Can you work these out from the model? Positions are in its coordinate system, mm. A direction names the side the tool comes from. Round coordinates to 2 decimals unless told otherwise and drop trailing zeros. Write each loop counter-clockwise with the first axis right and the second up, starting at its lowest first coordinate (ties: lowest second). Pieces come first, ordered by that corner, then holes. Notation, with made-up numbers: M 42.25,-39.5 L 91.25,-39.5 A21 ccw 91.25,-30.5 Z; hole C -35.75,-19.75 d9. An arc over 180 degrees is marked long. Answer as a JSON object with one key per item and string values. Group by question number.
1) Please list where these lines run through material, in increasing order: L1, parallel to Y at x = 0, z = 6.1; L2, parallel to Y at x = -2.5, z = 4; L3, parallel to X at y = 4.25, z = 7.5. Write a range as [from, to].
2) If we mould it in two halves opening along Y, with no side actions, what happens to faces 1 (the flat face through (0, -4, 8)), 2 (the flat face through (0, 4.75, 5)), 3 (the cylindrical face through (-0.75, 5.7, 5.97))? For each: +Y half, -Y half, draft (parallel to the pull), parting line (faces both ways), or undercut.
3) Suppose I cut it at A-A, the plane z = 7.5. Write out the boundary of the cut face in (x, y), and give its area (3 significant figures).
4) I'm going to push flat-ended pins straight in: pin 1 Ø4.5 at (x, y) = (0, 0) entering from +Z; pin 2 Ø6 at (x, y) = (1.5, -1) entering from +Z; pin 3 Ø1.5 at (x, y) = (3.5, 3.5) entering from -Z; pin 4 Ø1 at (x, z) = (2.5, 6) entering from -Y. Where does each tip first touch, or does it pass through?
5) On a 3-axis mill with a long thin cutter (end or side, diameter ignored), from which of +Z, -Z, +X, -X, +Y, -Y can I reach the whole of each face in a straight line? I mean faces 4 (the flat face through (-1, 4, 5)), 5 (the flat face through (0, 0, 0)). Say none if no direction works.
from build123d import *

# Parameters (mm, degrees)
F0_R     = 5.75
F1_DEPTH = 8
F2_DEPTH = 2
F3_R     = 4


with BuildPart() as f1:
    # F0 (on Top) → F1 (new body)
    with BuildSketch(Plane.XY):
        Circle(F0_R)
        with BuildLine():
            ThreePointArc((1, 3.614208), (2.984334, 2.270738), (3.75, 0))
            ThreePointArc((3.75, 0), (-2.270738, -2.984334), (-1, 3.614208))
            Line((-1, 3.614208), (-1, 4.75))
            Line((-1, 4.75), (1, 4.75))
            Line((1, 4.75), (1, 3.614208))
        make_face(mode=Mode.SUBTRACT)
    extrude(amount=F1_DEPTH)

    # F0 (on Top) → F2 (join)
    with BuildSketch(Plane.XY):
        with BuildLine():
            ThreePointArc((-1, 3.614208), (0, 3.75), (1, 3.614208))
            Line((1, 3.614208), (1, 4.75))
            Line((1, 4.75), (-1, 4.75))
            Line((-1, 4.75), (-1, 3.614208))
        make_face()
        with BuildLine():
            Line((1, 2.75), (1, 3.614208))
            ThreePointArc((1, 3.614208), (0, 3.75), (-1, 3.614208))
            Line((-1, 3.614208), (-1, 2.75))
            Line((-1, 2.75), (1, 2.75))
        make_face()
        with BuildLine():
            ThreePointArc((-1, 3.614208), (-2.270738, -2.984334), (3.75, 0))
            ThreePointArc((3.75, 0), (2.984334, 2.270738), (1, 3.614208))
            Line((1, 3.614208), (1, 2.75))
            Line((1, 2.75), (-1, 2.75))
            Line((-1, 2.75), (-1, 3.614208))
        make_face()
    extrude(amount=F2_DEPTH)

    # F3
    f3_edges = [f1.edges().sort_by_distance(p)[0] for p in [
        (-5.75, 0, 0),
    ]]
    fillet(f3_edges, radius=F3_R)


solid = f1.part
Results:
{
 "1": {"L1": "[-5.75, -3.75], [4.75, 5.75]", "L2": "[-5.18, -2.8], [2.8, 5.18]", "L3": "[-3.87, -1], [1, 3.87]"},
 "2": {"face 1": "draft", "face 2": "undercut", "face 3": "parting line"},
 "3": {"outline": "C 0,0 d11.5; hole M -1,3.61 A3.75 ccw long 1,3.61 L 1,4.75 L -1,4.75 Z", "area": "57.6 mm^2"},
 "4": {"pin 1": "z = 2", "pin 2": "z = 8", "pin 3": "z = 0.84", "pin 4": "y = -5.39"},
 "5": {"face 4": "+Z", "face 5": "-Z, +X, -X, +Y, -Y"}
}
